from build123d import *

# Parameters (mm, degrees)
SKIZZE1_W                       = 220
SKIZZE1_H                       = 220
AUFSATZ_LINEAR_AUSTRAGEN1_DEPTH = 10
SKIZZE3_R                       = 4.5
SCHNITT_LINEAR_AUSTRAGEN1_DEPTH = 156.884572681
SKIZZE4_R                       = 3.4
SCHNITT_LINEAR_AUSTRAGEN2_DEPTH = 156.884572681


with BuildPart() as part:
    # Skizze1 → Aufsatz-Linear austragen1 (new body)
    with BuildSketch(Plane.XY):
        Rectangle(SKIZZE1_W, SKIZZE1_H)
    extrude(amount=AUFSATZ_LINEAR_AUSTRAGEN1_DEPTH)

    # Skizze3 → Schnitt-Linear austragen1 (cut, through all)
    with BuildSketch(Plane.XY.offset(10)):
        with Locations((100, 0)):
            Circle(SKIZZE3_R)
        with Locations((0, -100)):
            Circle(SKIZZE3_R)
        with Locations((-100, 0)):
            Circle(SKIZZE3_R)
        with Locations((0, 100)):
            Circle(SKIZZE3_R)
    extrude(amount=-SCHNITT_LINEAR_AUSTRAGEN1_DEPTH, mode=Mode.SUBTRACT)

    # Skizze4 → Schnitt-Linear austragen2 (cut, through all)
    with BuildSketch(Plane.XY.offset(10)):
        with Locations((40, 70)):
            Circle(SKIZZE4_R)
        with Locations(Location((-40, 70, 0), (0, 0, 180))):
            Circle(SKIZZE4_R)
        with Locations(Location((40, -70, 0), (0, 0, 180))):
            Circle(SKIZZE4_R)
        with Locations((-40, -70)):
            Circle(SKIZZE4_R)
    extrude(amount=-SCHNITT_LINEAR_AUSTRAGEN2_DEPTH, mode=Mode.SUBTRACT)


solid = part.part
The listing builds one solid part. Answer for the finished solid, in the listing's coordinates (mm). Coordinates: 2 decimals unless noted, no trailing zeros. Order: outer loops, then holes, each group sorted by start corner. A loop starts at its lowest first (then second) coordinate and runs counter-clockwise, first axis right, second up.
Q1. A cutting plane is placed at B-B, the plane y = 100. Write down the section's boundary in (x, z), and give its area (3 significant figures).
Q2. A cutting plane is placed at A-A, the plane x = 0. Write down the section's boundary in (y, z).
Q3. A cutting plane is placed at D-D, the plane y = -70. Write down the section's boundary in (x, z), and give its area (3 significant figures).
Q4. Consider line 1 (Y direction, x = 40, z = 3.5); line 2 (X direction, y = 68, z = 1.75); line 3 (Y direction, x = 3.5, z = 6.25). Determine where each line is inside the solid, lowest interval first.
Q5. For a pull along X with two mould halves and no side action, classify faces 1 (the face through (-2, -110, 5)), 2 (the face through (41.6, 67, 5.1)), 3 (the face through (110, -2, 5)) as pulls with the +X half, pulls with the -X half, needs draft (parallel to the pull), parting line crosses it, or undercut.
Q6. Given P1, Ø6, axis at x = 40, y = -70, coming from the -Z side, flat-ended and moving along its own axis, determine where the tip first touches the part or whether it passes through.
Answers follow:
1. outline: (-110, 0) - (-4.5, 0) - (-4.5, 10) - (-110, 10) - close; (4.5, 0) - (110, 0) - (110, 10) - (4.5, 10) - close
1. area: 2,110 mm2
2. outline: (-110, 0) - (-104.5, 0) - (-104.5, 10) - (-110, 10) - close; (-95.5, 0) - (95.5, 0) - (95.5, 10) - (-95.5, 10) - close; (104.5, 0) - (110, 0) - (110, 10) - (104.5, 10) - close
3. outline: (-110, 0) - (-43.4, 0) - (-43.4, 10) - (-110, 10) - close; (-36.6, 0) - (36.6, 0) - (36.6, 10) - (-36.6, 10) - close; (43.4, 0) - (110, 0) - (110, 10) - (43.4, 10) - close
3. area: 2,060 mm2
4. line 1: y = -110 to -73.4, -66.6 to 66.6, 73.4 to 110
4. line 2: x = -110 to -42.75, -37.25 to 37.25, 42.75 to 110
4. line 3: y = -110 to -102.83, -97.17 to 97.17, 102.83 to 110
5. face 1: needs draft
5. face 2: undercut
5. face 3: pulls with the +X half
6. P1: passes through
